Geometry check sheet. Reference: the model listing, model coordinates, mm. A direction names the side the tool comes from. Coordinates: 2 decimals unless noted, no trailing zeros. Loops run counter-clockwise (first coordinate to the right, second up) from the corner with the lowest first, then second, coordinate; pieces in that order, holes last.
Autodesk Inventor part; units mm, degrees
ref_plane "Work Plane1" through (15, 0, 0) normal (1, 0, 0) x (0, 1, 0)
ref_plane "Work Plane2" through (52.6524, -10, -0.5) normal (0, 0, -1) x (-1, 0, 0)
ref_plane "Work Plane3" through (15, -10, 0.5) normal (0, 0, 1) x (1, 0, 0)
sketch "Sketch1" plane through (0, 0, 0) normal (0, 0, 1) x (1, 0, 0)
  line L0 (-336.1151, 0) -> (336.1151, 0) construction
  line L1 (15, 0) -> (50, 0) construction
  arc A0 (118.85, 219.94) -> (113.6034, 240) centre (-43.6266, 188.1614) ccw
  spline S0 degree 3 poles (118.85, 219.94) (128.5526, 163.9297) (111.383, 35.0272) (50, 0) knots 0 0 0 0 1 1 1 1
  line L2 (15, -15) -> (-15, -15)
  line L3 (-15, -15) -> (-15, 15)
  line L4 (-15, 15) -> (15, 15)
  line L5 (15, 15) -> (15, -15)
  line L6 (15, -15) -> (-15, 15) construction
  line L7 (-15, -15) -> (15, 15) construction
  line L8 (-32.5, -4.15) -> (32.5, -4.15) construction
  line L9 (32.5, -4.15) -> (32.5, 4.15) construction
  line L10 (32.5, 4.15) -> (-32.5, 4.15) construction
  line L11 (-32.5, 4.15) -> (-32.5, -4.15) construction
  line L12 (-32.5, -4.15) -> (32.5, 4.15) construction
  line L13 (32.5, -4.15) -> (-32.5, 4.15) construction
  arc A1 (15, 0) -> (50, 0) centre (32.5, 54.6766) ccw
  arc A2 (0, 15) -> (0, 50) centre (-54.6766, 32.5) ccw
  spline S1 degree 3 poles (-219.94, 118.85) (-163.9297, 128.5526) (-35.0272, 111.383) (0, 50) knots 0 0 0 0 1 1 1 1
  arc A3 (-219.94, 118.85) -> (-240, 113.6034) centre (-188.1614, -43.6266) ccw
  arc A4 (-15, 0) -> (-50, 0) centre (-32.5, -54.6766) ccw
  spline S2 degree 3 poles (-118.85, -219.94) (-128.5526, -163.9297) (-111.383, -35.0272) (-50, 0) knots 0 0 0 0 1 1 1 1
  arc A5 (-118.85, -219.94) -> (-113.6034, -240) centre (43.6266, -188.1614) ccw
  arc A6 (0, -15) -> (0, -50) centre (54.6766, -32.5) ccw
  spline S3 degree 3 poles (219.94, -118.85) (163.9297, -128.5526) (35.0272, -111.383) (0, -50) knots 0 0 0 0 1 1 1 1
  arc A7 (219.94, -118.85) -> (240, -113.6034) centre (188.1614, 43.6266) ccw
  point P0 (0, 0)
  point P1 (96.03, 57.2611)
  point P2 (119.66, 152.26)
  point P3 (119.6553, 152.2584)
  point P4 (0, 0)
  point P5 (-152.2584, 119.6553)
  point P6 (-57.2611, 96.03)
  point P7 (-15, 0)
  point P8 (-119.6553, -152.2584)
  point P9 (-96.03, -57.2611)
  point P10 (0, -15)
  point P11 (240, -113.6034)
  point P12 (152.2584, -119.6553)
  point P13 (57.2611, -96.03)
  point P14 (-15, 0)
  point P15 (-152.2584, 119.6553)
  point P16 (-57.2611, 96.03)
  point P17 (-119.6553, -152.2584)
  point P18 (-96.03, -57.2611)
  point P19 (152.2584, -119.6553)
  point P20 (57.2611, -96.03)
  dimension "d0" = 50
  dimension "d1" = 57.2611
  dimension "d2" = 96.03
  dimension "d3" = 119.66
  dimension "d6" = 118.85
  dimension "d12" = 240
  dimension "d38" = 65
  dimension "d39" = 8.3
  dimension "d61" = 360
sketch "Sketch2" plane through (0, 0, 0) normal (1, 0, 0) x (0, 1, 0)
  point P0 (0, 0)
  point P1 (0, 0)
  point P2 (240, 0)
ref_plane "Work Plane1" through (15, 0, 0) normal (1, 0, 0) x (0, 1, 0)
sketch "Sketch3" plane through (15, 0, 0) normal (1, 0, 0) x (0, 1, 0)
  line L0 (-10, -0.5) -> (10, -0.5)
  line L1 (10, -0.5) -> (10, 0.5)
  line L2 (10, 0.5) -> (-10, 0.5)
  line L3 (-10, 0.5) -> (-10, -0.5)
  line L4 (-10, -0.5) -> (10, 0.5) construction
  line L5 (10, -0.5) -> (-10, 0.5) construction
  point P0 (0, 0)
  dimension "d8" = 20
  dimension "d9" = 1
ref_plane "Work Plane2" through (52.6524, -10, -0.5) normal (0, 0, -1) x (-1, 0, 0)
sketch "Sketch4" plane through (52.6524, -10, -0.5) normal (0, 0, -1) x (-1, 0, 0)
  point P0 (52.6524, 10)
  point P1 (2.6524, 10)
  point P2 (-43.3776, 67.2611)
  point P3 (-67.0076, 162.26)
  point P4 (-66.1976, 229.94)
ref_plane "Work Plane3" through (15, -10, 0.5) normal (0, 0, 1) x (1, 0, 0)
sketch "Sketch5" plane through (15, -10, 0.5) normal (0, 0, 1) x (1, 0, 0)
  line L0 (17.5, 14.15) -> (-47.5, 14.15) construction
  line L1 (-47.5, 5.85) -> (17.5, 5.85) construction
  line L2 (-47.5, 14.15) -> (-47.5, 5.85) construction
  line L3 (17.5, 5.85) -> (17.5, 14.15) construction
  line L4 (0, -5) -> (20, -5)
  line L5 (20, -5) -> (20, 25)
  line L6 (20, 25) -> (0, 25)
  line L7 (0, 25) -> (0, -5)
  line L8 (0, 14.15) -> (20, 25) construction
  line L9 (20, 14.15) -> (0, 25) construction
  line L10 (0, -5) -> (20, 5.85) construction
  line L11 (20, -5) -> (0, 5.85) construction
  line L12 (10, 19.575) -> (10, 0.425) construction
  point P0 (-15, 10)
  point P1 (0, 25)
  point P2 (-30, 25)
  point P3 (-30, -5)
  dimension "d40" = 20
  dimension "d41" = 30
ref_plane "Work Plane5" through (15, 15, 0.5) normal (0, 0, 1) x (1, 0, 0)
sketch "Sketch6" plane through (15, 15, 0.5) normal (0, 0, 1) x (1, 0, 0)
  circle A0 centre (81.03, 42.2611) radius 6.8
  circle A1 centre (103.85, 204.94) radius 6.8
  circle A2 centre (104.66, 137.26) radius 6.8
  circle A3 centre (35, -15) radius 6.8
  arc A4 (113.2428, 206.6719) -> (106.6941, 230.8772) centre (-58.6266, 173.1614) ccw
  line L0 (90.5128, 219.1228) -> (106.6941, 230.8772)
  arc A5 (94.5125, 203.2183) -> (90.5128, 219.1228) centre (-58.6266, 173.1614) ccw
  arc A6 (20, -8.1753) -> (29.677, -6.6675) centre (17.5, 39.6766) ccw
  line L1 (20, -8.1753) -> (20, 0)
  line L2 (20, 0) -> (0, 0)
  line L3 (0, 0) -> (0, -15)
  line L4 (-1.9583, -24.4011) -> (0, -15)
  arc A7 (-1.9583, -24.4011) -> (0, -24.9633) centre (17.5, 39.6766) ccw
  line L5 (0, -24.9633) -> (0, -30)
  line L6 (0, -30) -> (20, -30)
  line L7 (20, -30) -> (20, -27.2437)
  arc A8 (20, -27.2437) -> (37.8217, -24.1325) centre (17.5, 39.6766) ccw
  circle A9 centre (10, -24.575) radius 3
  circle A10 centre (10, -5.425) radius 3
  line L8 (0, -15) -> (0, 0)
  line L9 (0, 0) -> (-1.9583, 0)
  line L10 (-1.9583, 0) -> (-1.9583, -30)
  line L11 (-1.9583, -30) -> (0, -30)
  line L12 (0, -30) -> (0, 0)
  point P0 (-15, -15)
ref_plane "Work Plane4" through (15, 15, 0.5) normal (0, 0, 1) x (1, 0, 0)
sketch "Sketch7" plane through (15, 15, 0.5) normal (0, 0, 1) x (1, 0, 0)
  line L0 (-50, -30) -> (20, -30)
  line L1 (20, -30) -> (20, 0)
  line L2 (20, 0) -> (-50, 0)
  line L3 (-50, 0) -> (-50, -30)
  line L4 (-16, -30) -> (-14, -30)
  line L5 (-14, 0) -> (-16, 0)
  line L6 (20, -20) -> (20, -10)
  line L7 (-50, -10) -> (-50, -20)
  line L8 (20, 0) -> (20, -30)
  line L9 (20, -30) -> (0, -30)
  line L10 (-50, 0) -> (-30, 0)
  line L11 (-30, -30) -> (-50, -30)
  line L12 (-50, -30) -> (-50, 0)
  line L13 (20, -10) -> (20, 0)
  line L14 (20, 0) -> (0, 0)
  line L15 (0, -30) -> (20, -30)
  line L16 (20, -20) -> (20, -30)
  line L17 (20, -30) -> (0, -30)
  line L18 (-30, -30) -> (-16, -30)
  circle A0 centre (10, -5.425) radius 3
  circle A1 centre (10, -24.575) radius 3
  line L19 (-50, -15) -> (20, -15) construction
  circle A2 centre (-40, -5.425) radius 3
  circle A3 centre (-40, -24.575) radius 3
  line L20 (-48.7, -19.15) -> (18.7, -19.15) construction
  line L21 (-48.7, -10.85) -> (-48.7, -15) construction
  line L22 (-48.7, -19.15) -> (18.7, -10.85) construction
  line L23 (18.7, -19.15) -> (-48.7, -10.85) construction
  line L24 (-15, -10.85) -> (-18.212, -6.8756)
  line L25 (-15, -10.85) -> (-11.788, -6.8756)
  line L26 (-50, -19.15) -> (-50, -10.85)
  line L27 (20, -19.15) -> (18.7, -19.15)
  line L28 (20, -10.85) -> (20, -19.15)
  line L29 (18.7, -10.85) -> (-11.788, -10.85) construction
  line L30 (-18.212, -10.85) -> (-48.7, -10.85) construction
  line L31 (-18.212, -6.8756) -> (-11.788, -6.8756)
  line L32 (-48.7, -15) -> (-49.61, -12.5368)
  line L33 (-48.7, -15) -> (-49.61, -17.4632)
  line L34 (-49.61, -17.4632) -> (-49.61, -12.5368)
  line L35 (-18.212, -6.8756) -> (-11.788, -6.8756)
  line L36 (-11.788, -6.8756) -> (-11.788, -10.85)
  line L37 (-11.788, -10.85) -> (-18.212, -10.85)
  line L38 (-18.212, -10.85) -> (-18.212, -6.8756)
  line L39 (-15, -19.15) -> (-18.212, -23.1244)
  line L40 (-15, -19.15) -> (-11.788, -23.1244)
  line L41 (-18.212, -23.1244) -> (-11.788, -23.1244)
  line L42 (-18.212, -23.1244) -> (-11.788, -23.1244)
  line L43 (-11.788, -23.1244) -> (-11.788, -19.15)
  line L44 (-11.788, -19.15) -> (-18.212, -19.15)
  line L45 (-18.212, -19.15) -> (-18.212, -23.1244)
  line L46 (-15, 0) -> (-15, -30) construction
  line L47 (-49.61, -12.5368) -> (-48.7, -12.5368)
  line L48 (-48.7, -12.5368) -> (-48.7, -17.4632)
  line L49 (-48.7, -17.4632) -> (-49.61, -17.4632)
  line L50 (-49.61, -17.4632) -> (-49.61, -12.5368)
  line L51 (18.7, -15) -> (19.61, -12.5368)
  line L52 (18.7, -15) -> (19.61, -17.4632)
  line L53 (19.61, -17.4632) -> (19.61, -12.5368)
  line L54 (19.61, -12.5368) -> (18.7, -12.5368)
  line L55 (18.7, -12.5368) -> (18.7, -17.4632)
  line L56 (18.7, -17.4632) -> (19.61, -17.4632)
  line L57 (19.61, -17.4632) -> (19.61, -12.5368)
  circle A4 centre (-24.575, -40) radius 3
  circle A5 centre (-5.425, -40) radius 3
  circle A6 centre (10, -24.575) radius 3
  circle A7 centre (10, -5.425) radius 3
  circle A8 centre (-5.425, 10) radius 3
  circle A9 centre (-24.575, 10) radius 3
  line L58 (-30, 20) -> (0, 20)
  line L59 (0, 20) -> (0, 0)
  line L60 (0, 0) -> (-30, 0)
  line L61 (-30, 0) -> (-30, 20)
  line L62 (-30, 20) -> (0, 0) construction
  line L63 (0, 20) -> (-30, 0) construction
  line L64 (-30, -50) -> (0, -50)
  line L65 (0, -50) -> (0, -30)
  line L66 (-30, -30) -> (-30, -50)
  line L67 (-30, -50) -> (0, -50)
  line L68 (0, -50) -> (0, -30)
  line L69 (0, -30) -> (-30, -30)
  line L70 (-30, -30) -> (-30, -50)
  point P0 (-15, -15)
  point P1 (-15, 10)
  dimension "d63" = 2
  dimension "d72" = 6
  dimension "d73" = 6
  dimension "d77" = 67.4
  dimension "d78" = 8.3
  dimension "d84" = 70
  dimension "d91" = 360
  dimension "d93" = 30
extrude "Extrusion7" add sketch "Sketch7" along normal blind 3 contours L3 L2 L1 L0 | L24 L31 L25 | L33 L34 L32 | L40 L41 L39 | L51 L53 L52
extrude "Extrusion8" add sketch "Sketch7" along normal blind 3 contours L61 L58 L59 L2
extrude "Extrusion9" add sketch "Sketch7" along normal blind 3 contours L0 L65 L64 L66
fillet "Fillet7" radius 4 12 edges at (15, 15, 2) (15, 35, 2) (35, 15, 2) (35, -15, 2) (15, -35, 2) (-15, -35, 2) (-15, -15, 2) (-35, -15, 2) (-35, 15, 2) (-15, 35, 2) (-15, 15, 2) (15, -15, 2)
sketch "Sketch8" plane through (15, 15, 3.5) normal (0, 0, 1) x (1, 0, 0)
  line L0 (-49.61, -12.5368) -> (-48.7, -12.5368) construction
  line L1 (19.61, -17.4632) -> (18.7, -17.4632) construction
  line L2 (-48.7, -12.5368) -> (18.7, -17.4632) construction
  line L3 (-48.7, -17.4632) -> (18.7, -12.5368) construction
  line L4 (-48.7, -12.5368) -> (18.7, -12.5368) construction
  line L5 (18.7, -12.5368) -> (18.7, -17.4632) construction
  line L6 (18.7, -17.4632) -> (-48.7, -17.4632) construction
  line L7 (-48.7, -17.4632) -> (-48.7, -12.5368) construction
  line L8 (-48.7, -12.5368) -> (-15, -12.5368) construction
  line L9 (-15, -12.5368) -> (-15, -17.4632) construction
  line L10 (-15, -17.4632) -> (-48.7, -17.4632) construction
  line L11 (-48.7, -17.4632) -> (-48.7, -12.5368) construction
  line L12 (-31.85, -17.4632) -> (-31.85, 4.3897) construction
  line L13 (-48.7, -15) -> (-15, -15) construction
  line L14 (-31.85, -6.5368) -> (-1.9543, -6.5368) construction
  line L15 (-48.7, -17.4632) -> (18.7, -17.4632)
  line L16 (18.7, -17.4632) -> (18.7, -12.5368)
  line L17 (18.7, -12.5368) -> (-48.7, -12.5368)
  line L18 (-48.7, -12.5368) -> (-48.7, -17.4632)
  point P0 (-25, -6.5368)
  point P1 (-25, -23.4632)
  point P2 (-5, -6.5368)
  point P3 (-5, -23.4632)
  dimension "d99" = 6
  dimension "d107" = 10
hole "Hole4" at (-10, 8.4632, 3.5) at (-10, -8.4632, 3.5) at (10, -8.4632, 3.5) at (10, 8.4632, 3.5) direction (0, 0, -1) diameter 5 end through all
sketch "Sketch9" plane through (15, 15, 3.5) normal (0, 0, 1) x (1, 0, 0)
  line L0 (-49.61, -12.5368) -> (-48.7, -12.5368)
  line L1 (-48.7, -15) -> (-49.61, -12.5368)
  line L2 (-49.61, -17.4632) -> (-48.7, -15)
  line L3 (-48.7, -15) -> (-48.7, -17.4632)
  line L4 (-48.7, -17.4632) -> (-49.61, -17.4632)
  line L5 (-48.7, -12.5368) -> (-48.7, -15)
  line L6 (18.7, -12.5368) -> (19.61, -12.5368)
  line L7 (19.61, -12.5368) -> (18.7, -15)
  line L8 (18.7, -15) -> (18.7, -12.5368)
  line L9 (18.7, -17.4632) -> (18.7, -15)
  line L10 (18.7, -15) -> (19.61, -17.4632)
  line L11 (19.61, -17.4632) -> (18.7, -17.4632)
  point P0 (-15, -15)
extrude "Extrusion10" add sketch "Sketch9" against normal blind 3
properties part number "underbrink_base_lite" material "Stainless Steel"
1) Access from +Z, -Z, +X, -X, +Y, -Y to the whole of each face (thin tool, end or side, straight path). Record for faces 1 (the flat face through (25, -15, 2)), 2 (the cylindrical face through (12.346, -23.851, 1.979)).
Data:
face 1: +Z, -Z, +X, -Y
face 2: +Z, -Z
2) Mould release check, pull along X, two halves, no side actions. Record for faces 3 (the flat face through (-25, 15, 2)), 4 (the cylindrical face through (24.35, 12.504, 1.979)), 5 (the cylindrical face through (-16.203, 16.141, 2.021)): +X half, -X half, draft (parallel to the pull), parting line (faces both ways), or undercut.
Data:
face 3: draft
face 4: undercut
face 5: -X half
3) Section check C-C on x = -10. Record the cut outline in (y, z), and give its area (3 significant figures).
Data:
outline: (-35, 0.5) - (-27.97, 0.5) - (-27.97, 3.5) - (-35, 3.5) - close; (-22.03, 0.5) - (-10.96, 0.5) - (-10.96, 3.5) - (-22.03, 3.5) - close; (-5.96, 0.5) - (5.96, 0.5) - (5.96, 3.5) - (-5.96, 3.5) - close; (10.96, 0.5) - (22.03, 0.5) - (22.03, 3.5) - (10.96, 3.5) - close; (27.97, 0.5) - (35, 0.5) - (35, 3.5) - (27.97, 3.5) - close
area: 144 mm2
4) Material ranges on probe 1 along Y at (x, z) = (-25, 2.3) (3 decimals); probe 2 along Y at (x, z) = (-10.5, 2.65); probe 3 along X at (y, z) = (-4.5, 2.95), recorded low to high.
Data:
probe 1: y = -15 to -12.575, -6.575 to 6.575, 12.575 to 15
probe 2: y = -35 to -27.85, -22.15 to -10.91, -6.01 to 6.01, 10.91 to 22.15, 27.85 to 35
probe 3: x = -35 to -3.21, -0.28 to 0.28, 3.21 to 35
5) Depth check by flat-ended pin: pin 1 (0.9 mm diameter, centred on x = -24, z = 2, fed in from -Y). Enter the tip coordinate at first touch or a pass-through.
Data:
pin 1: stops at y = -15
6) Section check A-A on y = -25. Record the cut outline in (x, z) (3 decimals).
Data:
outline: (-15, 0.5) - (-12.575, 0.5) - (-12.575, 3.5) - (-15, 3.5) - close; (-6.575, 0.5) - (6.575, 0.5) - (6.575, 3.5) - (-6.575, 3.5) - close; (12.575, 0.5) - (15, 0.5) - (15, 3.5) - (12.575, 3.5) - close
